Can you work these out from the model? Positions are in its coordinate system, mm. A direction names the side the tool comes from. Give positions to 0.01 mm unless a question says otherwise; leave off trailing zeros. Order: outer loops, then holes, each group sorted by start corner. A loop starts at its lowest first (then second) coordinate and runs counter-clockwise, first axis right, second up. Notation, with made-up numbers: (9, -11.5) - (32, -11.5) arc R18 ccw to (32, 3.5) - close; hole circle Ø6 at (86.25, 24.25). An arc over 180 degrees is marked (long way). Write each question's results on one line, items separated by ' | '. Start each with the question number.
from build123d import *

# Parameters (mm, degrees)
F0_R     = 7.9375
F1_DEPTH = 2.9718
F3_DEPTH = 2.9718


# Not quite as in the source:
# - a feature names something its author has since deleted; it is built from what else it names


with BuildPart() as f1:
    # F0 (on Top) → F1 (new body)
    with BuildSketch(Plane.XY):
        with BuildLine():
            ThreePointArc((-12.7, 0), (0, -12.7), (12.7, 0))
            ThreePointArc((12.7, 0), (0, 12.7), (-12.7, 0))
        make_face()
        Circle(F0_R, mode=Mode.SUBTRACT)
        with BuildLine():
            Line((12.7, -12.7), (12.7, 0))
            ThreePointArc((12.7, 0), (0, -12.7), (-12.7, 0))
            Line((-12.7, 0), (-12.7, -12.7))
            ThreePointArc((-12.7, -12.7), (0, -25.4), (12.7, -12.7))
        make_face()
    extrude(amount=-F1_DEPTH)

    # F2 (on face) → F3 (cut, through all)
    with BuildSketch(Plane.XY):
        with BuildLine():
            Line((12.7, -11.1125), (-1.4859, -11.1125))
            Line((-1.4859, -11.1125), (-1.4859, -17.4625))
            Line((-1.4859, -17.4625), (1.4859, -17.4625))
            Line((1.4859, -17.4625), (1.4859, -17.145))
            Line((1.4859, -17.145), (11.7732150983, -17.4625))
            ThreePointArc((11.7732150983, -17.4625), (12.4661508042, -15.1259192332), (12.7, -12.7))
            Line((12.7, -12.7), (12.7, -11.1125))
        make_face()
    extrude(amount=-F3_DEPTH, mode=Mode.SUBTRACT)


solid = f1.part
Q1. Which directions (+Z, -Z, +X, -X, +Y, -Y) give clear straight access to the entire face, cutting with the end or side of a thin tool? Please do faces 1 (the flat face through (6, -11.112, -1)), 2 (the flat face through (0, -10, 0)).
Q2. If I drill on probe 1 along Y at (x, z) = (0, -1.85); probe 2 along Y at (x, z) = (5, -2.55); probe 3 along X at (y, z) = (6.5, -0.9), over which ranges is the centre line in solid material (lowest first)? Write a range as from..to.
Q3. Thinking about a two-plate mould opening in Y: for faces 3 (the flat face through (0, -17.462, -1)), 4 (the cylindrical face through (-2.666, -25.117, -1.465)), 5 (the flat face through (0, -10, -2.972)), which applies, released by +Y, released by -Y, zero draft, split by the parting line, or undercut?
Q4. If we section it at B-B (x = 0): Please give me the cut outline in (y, z).
Q5. If we section it at C-C (y = 5): Please give me the cut outline in (x, z), plus the area to 3 significant figures.
Q6. Will this pin go through, and if not, where does the flat tip stop? P1, Ø1.5, axis at x = -7, z = -0.5, coming from the +Y side.
Q7. If we section it at D-D (y = -0.5): Please give me the cut outline in (x, z).
Findings below:
1) face 1: +Z, -Z, +X | face 2: +Z, +X, -X, +Y, -Y
2) probe 1: y = -25.4..-17.46, -11.11..-7.94, 7.94..12.7 | probe 2: y = -24.37..-17.25, -11.11..-6.16, 6.16..11.67 | probe 3: x = -10.91..-4.56, 4.56..10.91
3) face 3: undercut | face 4: released by -Y | face 5: zero draft
4) outline: (-25.4, -2.97) - (-17.46, -2.97) - (-17.46, 0) - (-25.4, 0) - close; (-11.11, -2.97) - (-7.94, -2.97) - (-7.94, 0) - (-11.11, 0) - close; (7.94, -2.97) - (12.7, -2.97) - (12.7, 0) - (7.94, 0) - close
5) outline: (-11.67, -2.97) - (-6.16, -2.97) - (-6.16, 0) - (-11.67, 0) - close; (6.16, -2.97) - (11.67, -2.97) - (11.67, 0) - (6.16, 0) - close | area: 32.7 mm2
6) P1: stops at y = 11.06
7) outline: (-12.7, -2.97) - (-7.92, -2.97) - (-7.92, 0) - (-12.7, 0) - close; (7.92, -2.97) - (12.7, -2.97) - (12.7, 0) - (7.92, 0) - close
